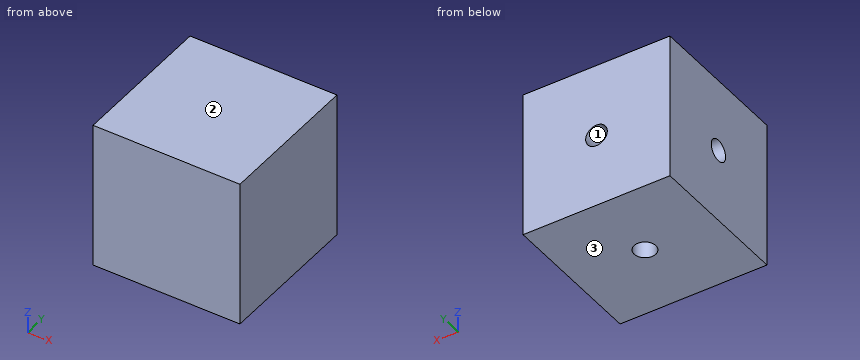
from build123d import *

# Parameters (mm, degrees)
F0_W          = 15.3162
F0_H          = 15.3162
F1_DEPTH      = 7.6581
F1_DEPTH_BACK = 7.6581
F3_D          = 2.2606
F3_DEPTH      = 14.605
F3_TIP        = 0.6791527577
F5_D          = 2.2606
F5_DEPTH      = 14.605
F5_TIP        = 0.6791527577
F7_D          = 2.2606
F7_DEPTH      = 14.605
F7_TIP        = 0.6791527577


with BuildPart() as f1:
    # F0 (on Top) → F1 (new body, two sides)
    with BuildSketch(Plane.XY) as f1_sk:
        Rectangle(F0_W, F0_H)
    extrude(amount=F1_DEPTH)
    extrude(f1_sk.sketch, amount=-F1_DEPTH_BACK)

    # F3
    with Locations(Plane(origin=(0, 7.6581, 0), x_dir=(-1, 0, 0), z_dir=(0, 1, 0))):
        with Locations((0, 0)):
            Hole(F3_D / 2, depth=F3_DEPTH)
            with Locations((0, 0, -(F3_DEPTH + F3_TIP / 2))):  # 118° drill point
                Cone(0, F3_D / 2, F3_TIP, mode=Mode.SUBTRACT)

    # F5
    with Locations(Plane(origin=(0, 0, -7.6581), x_dir=(1, 0, 0), z_dir=(0, 0, -1))):
        with Locations((0, 0)):
            Hole(F5_D / 2, depth=F5_DEPTH)
            with Locations((0, 0, -(F5_DEPTH + F5_TIP / 2))):  # 118° drill point
                Cone(0, F5_D / 2, F5_TIP, mode=Mode.SUBTRACT)

    # F7
    with Locations(Plane(origin=(-7.6581, 0, 0), x_dir=(0, -1, 0), z_dir=(-1, 0, 0))):
        with Locations((0, 0)):
            Hole(F7_D / 2, depth=F7_DEPTH)
            with Locations((0, 0, -(F7_DEPTH + F7_TIP / 2))):  # 118° drill point
                Cone(0, F7_D / 2, F7_TIP, mode=Mode.SUBTRACT)


solid = f1.part
The model under review builds one solid part; all positions refer to its coordinate system, in mm. Face numbers are marked on the shaded views. Round coordinates to 2 decimals unless told otherwise and drop trailing zeros. Order: outer loops, then holes, each group sorted by start corner. A loop starts at its lowest first (then second) coordinate and runs counter-clockwise, first axis right, second up. Notation, with made-up numbers: (50.25, 79.25) -> (83.25, 79.25) arc R30 cw to (83.25, 108.25) -> close; hole circle Ø8 at (4, -3). An arc over 180 degrees is marked (long way). Use CSV: the item, a comma, the result in double quotes. Start each with the question number.
(1) Consider section A-A on z = 4.5. Write out the cut boundary in (x, y), and give its area (3 significant figures).
(2) Wall thickness on probe 1 along Y at (x, z) = (0, 5): over which ranges is the line inside the solid? List them lowest first. Write a range as from..to.
(3) Mouldability with a two-part tool opening along Z and no side actions: class the marked faces 1, 2 and 3 as pulls with the +Z half, pulls with the -Z half, needs draft (parallel to the pull), parting line crosses it, or undercut.
Responses:
1,outline,"(-7.66, -7.66) -> (7.66, -7.66) -> (7.66, 7.66) -> (-7.66, 7.66) -> close; hole circle Ø2.26 at (0, 0)"
1,area,"231 mm²"
2,probe 1,"-7.66..-1.13, 1.13..7.66"
3,face 1,"undercut"
3,face 2,"pulls with the +Z half"
3,face 3,"pulls with the -Z half"
